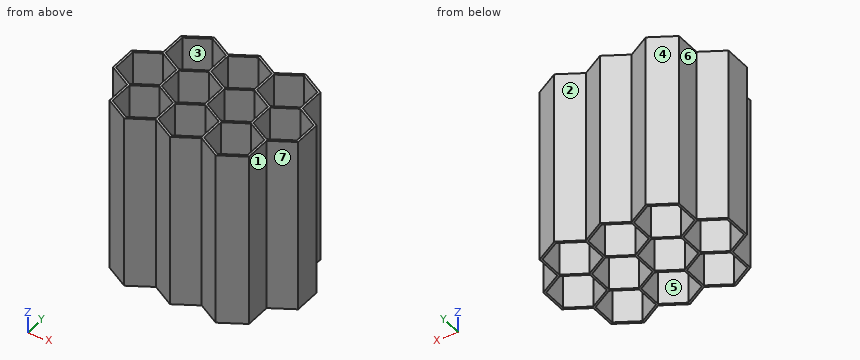
```python
from build123d import *

# Parameters (mm, degrees)
F1_DEPTH = 120
F3_DEPTH = 120.001


with BuildPart() as f1:
    # F0 (on Top) → F1 (new body)
    with BuildSketch(Plane.XY):
        Polygon((-35.93138, 37.175638), (-51.68138, 46.268904), (-68.18138, 36.742625), (-68.18138, 18.683001), (-84.041286, 9.526279), (-84.041286, -9.526279), (-68.18138, -18.683001), (-68.18138, -36.742625), (-51.68138, -46.268904), (-35.93138, -37.175638), (-20.18138, -46.268904), (-4.43138, -37.175638), (11.31862, -46.268904), (27.81862, -36.742625), (27.81862, -18.556092), (43.458714, -9.526279), (43.458714, 9.526279), (27.81862, 18.556092), (27.81862, 36.742625), (11.31862, 46.268904), (-4.43138, 37.175638), (-20.18138, 46.268904), align=None)
    extrude(amount=F1_DEPTH)

    # F2 (on face) → F3 (cut, through all)
    with BuildSketch(Plane.XY.offset(120)):
        Polygon((-51.68138, 44.536854), (-66.68138, 35.8766), (-66.68138, 18.556092), (-51.68138, 9.895837), (-36.68138, 18.556092), (-36.68138, 35.8766), align=None)
        Polygon((-67.541286, -17.320508), (-52.541286, -8.660254), (-52.541286, 8.660254), (-67.541286, 17.320508), (-82.541286, 8.660254), (-82.541286, -8.660254), align=None)
        Polygon((-51.68138, -44.536854), (-36.68138, -35.8766), (-36.68138, -18.556092), (-51.68138, -9.895837), (-66.68138, -18.556092), (-66.68138, -35.8766), align=None)
        Polygon((-20.18138, 9.895837), (-5.18138, 18.556092), (-5.18138, 35.8766), (-20.18138, 44.536854), (-35.18138, 35.8766), (-35.18138, 18.556092), align=None)
        Polygon((-5.18138, -18.556092), (-20.18138, -9.895837), (-35.18138, -18.556092), (-35.18138, -35.8766), (-20.18138, -44.536854), (-5.18138, -35.8766), align=None)
        Polygon((11.31862, 9.895837), (26.31862, 18.556092), (26.31862, 35.8766), (11.31862, 44.536854), (-3.68138, 35.8766), (-3.68138, 18.556092), align=None)
        Polygon((26.31862, -18.556092), (11.31862, -9.895837), (-3.68138, -18.556092), (-3.68138, -35.8766), (11.31862, -44.536854), (26.31862, -35.8766), align=None)
        Polygon((-21.041286, -8.660254), (-21.041286, 8.660254), (-36.041286, 17.320508), (-51.041286, 8.660254), (-51.041286, -8.660254), (-36.041286, -17.320508), align=None)
        Polygon((10.458714, -8.660254), (10.458714, 8.660254), (-4.541286, 17.320508), (-19.541286, 8.660254), (-19.541286, -8.660254), (-4.541286, -17.320508), align=None)
        Polygon((41.958714, -8.660254), (41.958714, 8.660254), (26.958714, 17.320508), (11.958714, 8.660254), (11.958714, -8.660254), (26.958714, -17.320508), align=None)
    extrude(amount=-F3_DEPTH, mode=Mode.SUBTRACT)


solid = f1.part
```
Geometry: final body of the model. Coordinates: model frame, mm. Face numbers are marked on the shaded views. A direction names the side the tool comes from. Give positions to 0.01 mm unless a question says otherwise; leave off trailing zeros. Loops run counter-clockwise (first coordinate to the right, second up) from the corner with the lowest first, then second, coordinate; pieces in that order, holes last. Notation, with made-up numbers: (23, 16.5) -> (55, 16.5) arc R34 ccw to (55, 49.5) -> close; hole circle Ø8 at (44, 86). An arc over 180 degrees is marked (long way). Use one line per item in the form item = value.
Item 1: Section query D-D on y = -12. Give the number of separate pieces and of enclosed holes in the cut face, and give its area (3 significant figures).
A:
separate_pieces = 8
enclosed_holes = 0
area = 2,800 mm^2
Item 2: Pin query (flat end, axial travel): P1, Ø19, axis at y = 26, z = 83, coming from the -X side; P2, Ø5.5, axis at y = 30, z = 43, coming from the +X side; P3, Ø5.5, axis at y = -27.5, z = 82, coming from the -X side; P4, Ø12, axis at x = -25.5, y = -25.5, coming from the +Z side. Return the tip coordinate at first contact, or that it passes through.
A:
P1 = -71.96
P2 = 27.82
P3 = -68.18
P4 = through
Item 3: Line query: probe 1 along X at (y, z) = (27, 67); probe 2 along X at (y, z) = (-1, 24.5); probe 3 along Y at (x, z) = (17.5, 83.5). Output: solid intervals per line, ascending.
A:
probe_1 = -68.18 to -66.68, -36.68 to -35.18, -5.18 to -3.68, 26.32 to 27.82
probe_2 = -84.04 to -82.54, -52.54 to -51.04, -21.04 to -19.54, 10.46 to 11.96, 41.96 to 43.46
probe_3 = -42.7 to -40.97, -13.46 to -11.86, 11.86 to 13.46, 40.97 to 42.7
Item 4: Section query A-A on y = 33. Output: boundary loops of the cut face in (x, z), and give its area (3 significant figures).
A:
outline = (-68.18, 0) -> (-66.68, 0) -> (-66.68, 120) -> (-68.18, 120) -> close; (-36.68, 0) -> (-35.18, 0) -> (-35.18, 120) -> (-36.68, 120) -> close; (-5.18, 0) -> (-3.68, 0) -> (-3.68, 120) -> (-5.18, 120) -> close; (26.32, 0) -> (27.82, 0) -> (27.82, 120) -> (26.32, 120) -> close
area = 720 mm^2
Item 5: Draft query along X for the marked faces 5, 6 and 7. Return one class per face: pulls with the +X half, pulls with the -X half, needs draft (parallel to the pull), parting line crosses it, or undercut.
A:
face_5 = undercut
face_6 = pulls with the -X half
face_7 = pulls with the +X half
Item 6: Section query B-B on y = 2. Output: boundary loops of the cut face in (x, z), and give its area (3 significant figures).
A:
outline = (-84.04, 0) -> (-82.54, 0) -> (-82.54, 120) -> (-84.04, 120) -> close; (-52.54, 0) -> (-51.04, 0) -> (-51.04, 120) -> (-52.54, 120) -> close; (-21.04, 0) -> (-19.54, 0) -> (-19.54, 120) -> (-21.04, 120) -> close; (10.46, 0) -> (11.96, 0) -> (11.96, 120) -> (10.46, 120) -> close; (41.96, 0) -> (43.46, 0) -> (43.46, 120) -> (41.96, 120) -> close
area = 900 mm^2
Item 7: Section query C-C on x = 6.5. Output: boundary loops of the cut face in (y, z), and give its area (3 significant figures).
A:
outline = (-43.49, 0) -> (-41.75, 0) -> (-41.75, 120) -> (-43.49, 120) -> close; (-12.68, 0) -> (-10.95, 0) -> (-10.95, 120) -> (-12.68, 120) -> close; (10.95, 0) -> (12.68, 0) -> (12.68, 120) -> (10.95, 120) -> close; (41.75, 0) -> (43.49, 0) -> (43.49, 120) -> (41.75, 120) -> close
area = 831 mm^2
Item 8: Access query for the marked faces 1, 2, 3 and 4. Directions: +Z, -Z, +X, -X, +Y, -Y. A direction counts if a zero-diameter tool reaches every point of the face in a straight line with its end or side. Return the directions, or none.
A:
face_1 = +Z, -Z, +X, -Y
face_2 = +Z, -Z, +Y
face_3 = +Z, -Z
face_4 = +Z, -Z, -X, +Y
